Answer from the drawing. Dimensions are ordinates in mm from the lowest x, y and z of the part. A direction names the side the tool comes from. Coordinates: 2 decimals unless noted, no trailing zeros. Write each loop counter-clockwise with the first axis right and the second up, starting at its lowest first coordinate (ties: lowest second). Pieces come first, ordered by that corner, then holes. Notation, with made-up numbers: (-2, 84.5) -> (16, 84.5) arc R30 cw to (16, 117.5) -> close; hole circle Ø4 at (-11, 80.5). An arc over 180 degrees is marked (long way). Answer as a JSON object with one key per item and string values. Group by question number.
(1) Which of the six approach directions +Z, -Z, +X, -X, +Y, -Y give full straight-line access (tool end or side, diameter ignored) to the marked faces 1 and 2?
(2) Straight lines are drawn through the part: L1, parallel to Y at x = 2, z = 4.25; L2, parallel to Z at x = 4, y = 1.5 (3 decimals); L3, parallel to Z at x = 2.75, y = 9.25. For each, find the intervals that lie inside material, in ascending order.
(3) Find section C-C (y = 1.5). Give the vertices of the cut face in (x, z) (3 decimals).
(4) Find section A-A (z = 4). Give the vertices of the cut face in (x, y) (3 decimals), then the cut area to 3 significant figures.
(5) Find section B-B (x = 4). Give the vertices of the cut face in (y, z) (3 decimals), then the cut area to 3 significant figures.
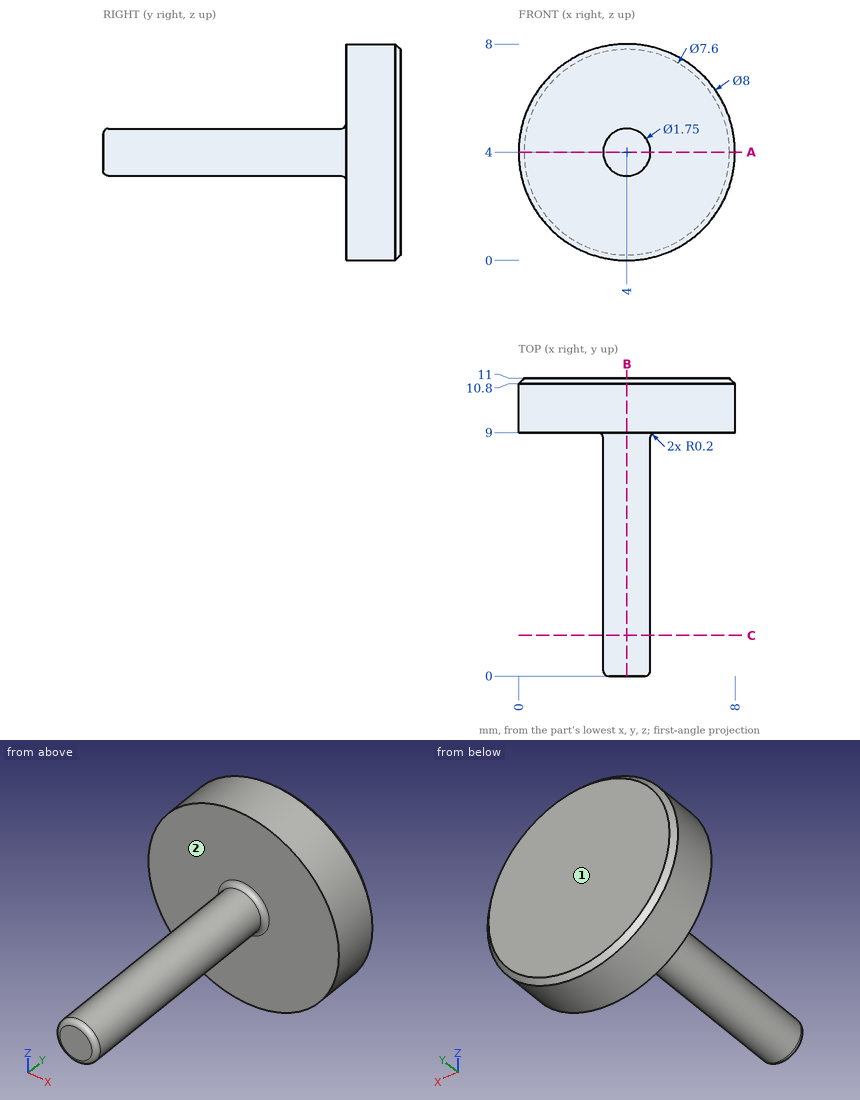
Results below:
{
 "1": {"face 1": "+Z, -Z, +X, -X, +Y", "face 2": "-Y"},
 "2": {"L1": "y = 9 to 11", "L2": "z = 3.125 to 4.875", "L3": "z = 0.2 to 7.8"},
 "3": {"outline": "circle Ø1.75 at (4, 4)"},
 "4": {"outline": "(0, 9) -> (2.925, 9) arc R0.2 cw to (3.125, 8.8) -> (3.125, 0.2) arc R0.2 ccw to (3.325, 0) -> (4.675, 0) arc R0.2 ccw to (4.875, 0.2) -> (4.875, 8.8) arc R0.2 cw to (5.075, 9) -> (8, 9) -> (8, 10.8) -> (7.8, 11) -> (0.2, 11) -> (0, 10.8) -> close", "area": "31.7 mm2"},
 "5": {"outline": "(0, 3.325) arc R0.2 ccw to (0.2, 3.125) -> (8.8, 3.125) arc R0.2 cw to (9, 2.925) -> (9, 0) -> (10.8, 0) -> (11, 0.2) -> (11, 7.8) -> (10.8, 8) -> (9, 8) -> (9, 5.075) arc R0.2 cw to (8.8, 4.875) -> (0.2, 4.875) arc R0.2 ccw to (0, 4.675) -> close", "area": "31.7 mm2"}
}
